Source: CAD feature listing. Evaluate the final solid. Frame: model axes, mm. Round coordinates to 2 decimals unless told otherwise and drop trailing zeros. Write each loop counter-clockwise with the first axis right and the second up, starting at its lowest first coordinate (ties: lowest second). Pieces come first, ordered by that corner, then holes. Notation, with made-up numbers: M -7,-11.75 L 2,-11.75 A24 ccw 2,22.25 Z; hole C -22,-26 d4. An arc over 180 degrees is marked long. Use a Markdown table: item, result.
```python
from build123d import *

# Parameters (mm, degrees)
F0_R     = 64.516
F2_DEPTH = 8
F3_DEPTH = 8
F4_R     = 4.5
F5_DEPTH = 8


with BuildPart() as f2:
    # F0 (on Top) → F2 (new body)
    with BuildSketch(Plane.XY):
        Circle(F0_R)
    extrude(amount=F2_DEPTH)

    # F1 (on Top) → F3 (cut, through all)
    with BuildSketch(Plane.XY):
        with BuildLine():
            Line((-19, 20), (-19, 0))
            Line((-19, 0), (-19, -20))
            ThreePointArc((-19, -20), (-13.435029, -33.435029), (0, -39))
            ThreePointArc((0, -39), (13.435029, -33.435029), (19, -20))
            Line((19, -20), (19, 0))
            Line((19, 0), (19, 20))
            ThreePointArc((19, 20), (13.435029, 33.435029), (0, 39))
            ThreePointArc((0, 39), (-13.435029, 33.435029), (-19, 20))
        make_face()
        with BuildLine():
            Line((-24.5, -25.75), (-24.5, 0))
            Line((-24.5, 0), (-24.5, 25.75))
            ThreePointArc((-24.5, 25.75), (-27.75, 29), (-31, 25.75))
            Line((-31, 25.75), (-31, 0))
            Line((-31, 0), (-31, -25.75))
            ThreePointArc((-31, -25.75), (-27.75, -29), (-24.5, -25.75))
        make_face()
        with BuildLine():
            Line((24.5, 25.75), (24.5, 0))
            Line((24.5, 0), (24.5, -25.75))
            ThreePointArc((24.5, -25.75), (27.75, -29), (31, -25.75))
            Line((31, -25.75), (31, 0))
            Line((31, 0), (31, 25.75))
            ThreePointArc((31, 25.75), (27.75, 29), (24.5, 25.75))
        make_face()
    extrude(amount=F3_DEPTH, mode=Mode.SUBTRACT)

    # F4 (on face) → F5 (cut, through all)
    with BuildSketch(Plane.XY.offset(8)):
        with Locations((0, -55.832823)):
            Circle(F4_R)
        with Locations((-44.5, 33.720234)):
            Circle(F4_R)
        with Locations((44.5, 33.720234)):
            Circle(F4_R)
    extrude(amount=-F5_DEPTH, mode=Mode.SUBTRACT)


solid = f2.part
```
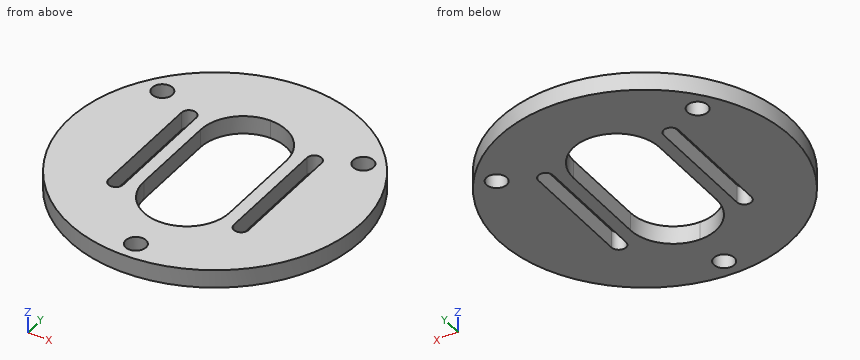
Q1. Section D-D on z = 2. Return loops of the section in (x, y), plus the area to 3 significant figures.
Results are:
| item | result |
|---|---|
| outline | C 0,0 d129.03; hole C -44.5,33.72 d9; hole M -31,-25.75 A3.25 ccw -24.5,-25.75 L -24.5,25.75 A3.25 ccw -31,25.75 Z; hole M -19,-20 A19 ccw 0,-39 A19 ccw 19,-20 L 19,20 A19 ccw 0,39 A19 ccw -19,20 Z; hole C 0,-55.83 d9; hole M 24.5,-25.75 A3.25 ccw 31,-25.75 L 31,25.75 A3.25 ccw 24.5,25.75 Z; hole C 44.5,33.72 d9 |
| area | 9,500 mm^2 |
Q2. Section C-C on x = 27.75. Return loops of the section in (y, z).
Results are:
| item | result |
|---|---|
| outline | M -58.24,0 L -29,0 L -29,8 L -58.24,8 Z; M 29,0 L 58.24,0 L 58.24,8 L 29,8 Z |
Q3. First-contact query: pin 1 Ø4 at (y, z) = (12, 5) entering from +X; pin 2 Ø2.5 at (y, z) = (-6, 3.5) entering from +X; pin 3 Ø4 at (x, y) = (-21.5, -29.5) entering from -Z; pin 4 Ø2 at (y, z) = (21, 7) entering from +X. Flat tips, straight axial feed; report the tip coordinate or a pass-through.
Results are:
| item | result |
|---|---|
| pin 1 | x = 63.74 |
| pin 2 | x = 64.34 |
| pin 3 | z = 0 |
| pin 4 | x = 61.34 |
Q4. Section B-B on x = 1.5. Return loops of the section in (y, z), plus the area to 3 significant figures.
Results are:
| item | result |
|---|---|
| outline | M -64.5,0 L -60.08,0 L -60.08,8 L -64.5,8 Z; M -51.59,0 L -38.94,0 L -38.94,8 L -51.59,8 Z; M 38.94,0 L 64.5,0 L 64.5,8 L 38.94,8 Z |
| area | 341 mm^2 |
Q5. Line query: L1, parallel to X at y = -4, z = 5; L2, parallel to Y at x = 3, z = 3.5; L3, parallel to X at y = 32, z = 5. Output: solid intervals per line, ascending.
Results are:
| item | result |
|---|---|
| L1 | -64.39 to -31, -24.5 to -19, 19 to 24.5, 31 to 64.39 |
| L2 | -64.45 to -59.19, -52.48 to -38.76, 38.76 to 64.45 |
| L3 | -56.02 to -48.66, -40.34 to -14.73, 14.73 to 40.34, 48.66 to 56.02 |
Q6. Section A-A on y = 0. Return loops of the section in (x, z).
Results are:
| item | result |
|---|---|
| outline | M -64.52,0 L -31,0 L -31,8 L -64.52,8 Z; M -24.5,0 L -19,0 L -19,8 L -24.5,8 Z; M 19,0 L 24.5,0 L 24.5,8 L 19,8 Z; M 31,0 L 64.52,0 L 64.52,8 L 31,8 Z |
